from build123d import *

# Parameters (mm, degrees)
F1_DEPTH = 8


with BuildPart() as f1:
    # F0 (on Top) → F1 (new body)
    with BuildSketch(Plane.XY):
        with BuildLine():
            ThreePointArc((-6, 0), (-1.2982424862, 5.8578636419), (5.4381888157, 2.5349758194))
            add(Edge.make_bspline(
                [(5.4381888157, 2.5349758194), (5.9168648922, 1.3048778647), (6.5712223704, 0.8342077495), (7.316287914, 0.5489782253), (7.3954237393, 0.5231885691)],
                knots=[0, 0, 0, 0, 0.5130903697, 0.5729750339, 0.5729750339, 0.5729750339, 0.5729750339], degree=3))
            ThreePointArc((7.3954237393, 0.5231885691), (7.6236703696, 0.4951548346), (7.8456981312, 0.5550387858))
            Line((7.8456981312, 0.5550387858), (9.3807354753, 1.30845808))
            Line((9.3807354753, 1.30845808), (9.5947175059, 1.4134836619))
            ThreePointArc((9.5947175059, 1.4134836619), (9.9019177362, 2.1346293669), (9.2336132629, 2.544253878))
            add(Edge.make_bspline(
                [(7.2891862958, 3.2966290579), (7.9620901058, 2.2604630582), (8.2498794852, 2.3761286058), (9.1349400628, 2.5281333533), (9.2336132629, 2.544253878)],
                knots=[0, 0, 0, 0, 0.4310159689, 0.4819722472, 0.4819722472, 0.4819722472, 0.4819722472], degree=3))
            ThreePointArc((7.2891862958, 3.2966290579), (-1.6861953673, 7.8202778201), (-8, 0))
            ThreePointArc((-8, 0), (-1.6861953673, -7.8202778201), (7.2891862958, -3.2966290579))
            add(Edge.make_bspline(
                [(7.2891862958, -3.2966290579), (7.9620901058, -2.2604630582), (8.2498794852, -2.3761286058), (9.1349400628, -2.5281333533), (9.2336132629, -2.544253878)],
                knots=[0, 0, 0, 0, 0.4310159689, 0.4819722472, 0.4819722472, 0.4819722472, 0.4819722472], degree=3))
            ThreePointArc((9.2336132629, -2.544253878), (9.9019177362, -2.1346293669), (9.5947175059, -1.4134836619))
            Line((9.5947175059, -1.4134836619), (9.3807354753, -1.30845808))
            Line((9.3807354753, -1.30845808), (7.8456981312, -0.5550387858))
            ThreePointArc((7.8456981312, -0.5550387858), (7.6236703696, -0.4951548346), (7.3954237393, -0.5231885691))
            add(Edge.make_bspline(
                [(5.4381888157, -2.5349758194), (5.9168648922, -1.3048778647), (6.5712223704, -0.8342077495), (7.316287914, -0.5489782253), (7.3954237393, -0.5231885691)],
                knots=[0, 0, 0, 0, 0.5130903697, 0.5729750339, 0.5729750339, 0.5729750339, 0.5729750339], degree=3))
            ThreePointArc((5.4381888157, -2.5349758194), (-1.2982424862, -5.8578636419), (-6, 0))
        make_face()
    extrude(amount=F1_DEPTH)


solid = f1.part
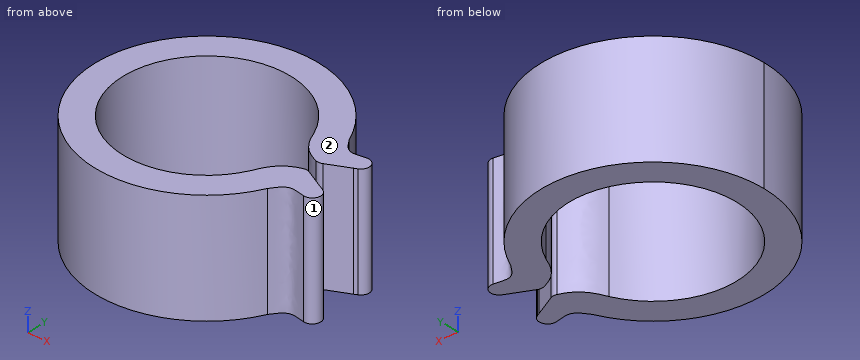
Verification items for the finished model (mm, model axes). Face numbers are marked on the shaded views. Round coordinates to 2 decimals unless told otherwise and drop trailing zeros. Loops run counter-clockwise (first coordinate to the right, second up) from the corner with the lowest first, then second, coordinate; pieces in that order, holes last. Notation, with made-up numbers: (68, -16.75) - (93, -16.75) arc R24 ccw to (93, 13.25) - close; hole circle Ø8 at (-12.75, -38.5). An arc over 180 degrees is marked (long way). Answer in a Markdown table with one row per item. Add a question column.
Q1. Gauge pin test, flat ends, axial feed: pin 1 (4 mm diameter, centred on x = -5, z = 3, fed in from -Y); pin 2 (1 mm diameter, centred on y = -4.5, z = 1.5, fed in from +X); pin 3 (1 mm diameter, centred on x = 8, y = 6, fed in from -Z); pin 4 (1.5 mm diameter, centred on x = 3, z = 1, fed in from +Y). Record the tip position at first contact, or that the pin passes through.
Q2. Section check A-A on x = 0. Enter the section's corners in (y, z).
Q3. Release check for a two-part mould opening along Y. For the marked faces 1 and 2 record: pulls with the +Y half, pulls with the -Y half, needs draft (parallel to the pull), parting line crosses it, or undercut.
Q4. Section check B-B on y = -4. Enter the section's corners in (x, z), plus the area to 3 significant figures.
Q5. Section check C-C on y = -6.5. Enter the section's corners in (x, z).
Q6. Material ranges on line 1 (Y direction, x = 0, z = 4.5); line 2 (Y direction, x = 5.25, z = 4); line 3 (X direction, y = 4, z = 1.5), recorded low to high.
Found:
| question | item | result |
|---|---|---|
| 1 | pin 1 | stops at y = -7.42 |
| 1 | pin 2 | stops at x = 6.93 |
| 1 | pin 3 | passes through |
| 1 | pin 4 | stops at y = 7.68 |
| 2 | outline | (-8, 0) - (-6, 0) - (-6, 8) - (-8, 8) - close; (6, 0) - (8, 0) - (8, 8) - (6, 8) - close |
| 3 | face 1 | undercut |
| 3 | face 2 | needs draft |
| 4 | outline | (-6.93, 0) - (-4.47, 0) - (-4.47, 8) - (-6.93, 8) - close; (4.47, 0) - (6.93, 0) - (6.93, 8) - (4.47, 8) - close |
| 4 | area | 39.3 mm² |
| 5 | outline | (-4.66, 0) - (4.66, 0) - (4.66, 8) - (-4.66, 8) - close |
| 6 | line 1 | y = -8 to -6, 6 to 8 |
| 6 | line 2 | y = -6.04 to -2.9, 2.9 to 6.04 |
| 6 | line 3 | x = -6.93 to -4.47, 4.47 to 6.93 |
